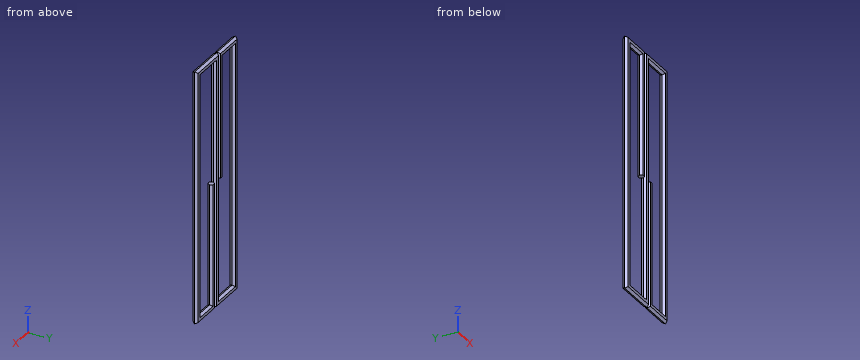
```python
from build123d import *


with BuildPart() as part:
    # Sweep2: sweep along a path in Sketch2
    with BuildLine(Plane(origin=(0, 0, 0), x_dir=(1, 0, 0), z_dir=(0, 1, 0))) as sweep2_path:
        Line((-25, 0), (-25, -475))
        Line((-25, -475), (-125, -475))
        Line((-125, -475), (-125, 475))
        Line((-125, 475), (0, 475))
        Line((0, 475), (0, -475))
        Line((0, -475), (125, -475))
        Line((125, -475), (125, 475))
        Line((125, 475), (25, 475))
        Line((25, 475), (25, 0))
    # Sketch3 → Sweep2 (sweep)
    with BuildSketch(Plane.XY):
        Polygon((36.547005384, 0), (30.773502692, 10), (19.226497308, 10), (13.452994616, 0), (19.226497308, -10), (30.773502692, -10), align=None)
    sweep(path=sweep2_path.line, transition=Transition.RIGHT)


solid = part.part
```
Geometry check sheet. Reference: the model listing, model coordinates, mm. Give positions to 0.01 mm unless a question says otherwise; leave off trailing zeros. Loops run counter-clockwise (first coordinate to the right, second up) from the corner with the lowest first, then second, coordinate; pieces in that order, holes last. Notation, with made-up numbers: M 88,69 L 147,69 A17 ccw 147,92 Z; hole C 80.5,-30.5 d7. An arc over 180 degrees is marked long. Write item = value, one per line.
(1) Gauge pin test, flat ends, axial feed: pin 1 Ø12 at (x, y) = (4.5, -8) entering from -Z; pin 2 Ø1.5 at (y, z) = (8, 13.5) entering from +X; pin 3 Ø1 at (y, z) = (-3, -36.5) entering from +X. Record the tip position at first contact, or that the pin passes through.
Answer below:
pin_1 = -485.39
pin_2 = 132.36
pin_3 = 135.1
(2) Sectioned sample at A-A, the plane x = -87.5. Record the cut outline in (y, z), plus the area to 3 significant figures.
Answer below:
outline = M -10,-480.77 L 0,-486.55 L 10,-480.77 L 10,-469.23 L 0,-463.45 L -10,-469.23 Z; M -10,469.23 L 0,463.45 L 10,469.23 L 10,480.77 L 0,486.55 L -10,480.77 Z
area = 693 mm2
(3) Sectioned sample at C-C, the plane y = 3.75. Record the cut outline in (x, z), plus the area to 3 significant figures.
Answer below:
outline = M -134.38,-484.38 L 9.38,-484.38 L 9.38,465.62 L 115.62,465.62 L 115.62,-465.62 L 34.38,-465.62 L 34.38,0 L 15.62,0 L 15.62,-484.38 L 134.38,-484.38 L 134.38,484.38 L -9.38,484.38 L -9.38,-465.62 L -115.62,-465.62 L -115.62,465.62 L -34.38,465.62 L -34.38,0 L -15.62,0 L -15.62,484.38 L -134.38,484.38 Z
area = 79,700 mm2
(4) Material ranges on line 1 (X direction, y = -8.75, z = 7.5); line 2 (X direction, y = 6, z = 272.5); line 3 (Z direction, x = 40, y = 3.75), recorded low to high. Write a range as [from, to].
Answer below:
line_1 = [-131.5, -118.5], [-31.5, -18.5], [-6.5, 6.5], [118.5, 131.5]
line_2 = [-133.08, -116.92], [-33.08, -16.92], [-8.08, 8.08], [116.92, 133.08]
line_3 = [-484.38, -465.62], [465.62, 484.38]
(5) Sectioned sample at B-B, the plane z = 52. Record the cut outline in (x, y).
Answer below:
outline = M -136.55,0 L -130.77,-10 L -119.23,-10 L -113.45,0 L -119.23,10 L -130.77,10 Z; M -36.55,0 L -30.77,-10 L -19.23,-10 L -13.45,0 L -19.23,10 L -30.77,10 Z; M -11.55,0 L -5.77,-10 L 5.77,-10 L 11.55,0 L 5.77,10 L -5.77,10 Z; M 113.45,0 L 119.23,-10 L 130.77,-10 L 136.55,0 L 130.77,10 L 119.23,10 Z
